from build123d import *
from OCP.BRepFilletAPI import BRepFilletAPI_MakeChamfer

# Parameters (mm, degrees)
SKETCH1_W           = 10.03
SKETCH1_H           = 7.51
BOSS_EXTRUDE1_DEPTH = 7.62
SKETCH2_W           = 2.03
SKETCH2_H           = 4.06
BOSS_EXTRUDE2_DEPTH = 0.89
CHAMFER1_SIZE       = 0.89
CHAMFER1_SIZE_2     = 0.238474781
SKETCH3_W           = 2.03
SKETCH3_H           = 4.06
CUT_EXTRUDE1_DEPTH  = 0.25
BOSS_EXTRUDE3_DEPTH = 0.28
LPATTERN1_COUNT     = 2
LPATTERN1_PITCH     = 2.54
FILLET1_R           = 0.1


with BuildPart() as part:
    # Sketch1 → Boss-Extrude1 (new body)
    with BuildSketch(Plane(origin=(0, 0, 0), x_dir=(1, 0, 0), z_dir=(0, 1, 0))):
        Rectangle(SKETCH1_W, SKETCH1_H)
    extrude(amount=BOSS_EXTRUDE1_DEPTH)

    # Sketch2 → Boss-Extrude2 (add)
    with BuildSketch(Plane(origin=(0, 7.62, 0), x_dir=(1, 0, 0), z_dir=(0, 1, 0))):
        with Locations((-1.015, 0)):
            Rectangle(SKETCH2_W, SKETCH2_H)
    extrude(amount=BOSS_EXTRUDE2_DEPTH)

    # Chamfer1
    chamfer1_edges_1 = [part.edges().sort_by_distance(p)[0] for p in [
        (-1.015, 8.51, -2.03),
    ]]
    chamfer1_side_1 = [part.faces().sort_by_distance(p)[0] for p in [
        (-1.015, 8.505230504, -2.03),
    ]]
    chamfer1_edges_2 = [part.edges().sort_by_distance(p)[0] for p in [
        (-1.015, 8.51, 2.03),
    ]]
    chamfer1_side_2 = [part.faces().sort_by_distance(p)[0] for p in [
        (-1.015, 8.505230504, 2.03),
    ]]
    chamfer1 = BRepFilletAPI_MakeChamfer(part.part.solid().wrapped)
    for e in chamfer1_edges_1:
        chamfer1.Add(CHAMFER1_SIZE - 0.0001, CHAMFER1_SIZE_2 - 0.0001, e.wrapped, chamfer1_side_1[0].wrapped)
    for e in chamfer1_edges_2:
        chamfer1.Add(CHAMFER1_SIZE - 0.0001, CHAMFER1_SIZE_2 - 0.0001, e.wrapped, chamfer1_side_2[0].wrapped)
    add(Compound.cast(chamfer1.Shape()), mode=Mode.REPLACE)  # a hair under: the kernel refuses the full size

    # Sketch3 → Cut-Extrude1 (cut)
    with BuildSketch(Plane(origin=(0, 7.62, 0), x_dir=(1, 0, 0), z_dir=(0, 1, 0))):
        with Locations((1.015, 0)):
            Rectangle(SKETCH3_W, SKETCH3_H)
    extrude(amount=-CUT_EXTRUDE1_DEPTH, mode=Mode.SUBTRACT)

    # Sketch4 → Boss-Extrude3 (add, symmetric)
    with BuildSketch(Plane.XY.offset(1.27)):
        Polygon((4.33, 0), (4, 0), (4, -1.85), (5.2, -1.85), (5.2, -1.52), (4.33, -1.52), align=None)
        Polygon((-4, -1.85), (-5.2, -1.85), (-5.2, -1.52), (-4.33, -1.52), (-4.33, 0), (-4, 0), align=None)
    boss_extrude3 = extrude(amount=BOSS_EXTRUDE3_DEPTH, both=True)

    # LPattern1: Boss-Extrude3 ×2
    with Locations(*[(0, 0, -i * LPATTERN1_PITCH) for i in range(1, LPATTERN1_COUNT)]):
        add(boss_extrude3)

    # Fillet1
    fillet1_edges = [part.edges().sort_by_distance(p)[0] for p in [
        (5.015, 7.62, 0),
        (0, 7.62, -3.755),
        (-5.015, 7.62, 0),
        (0, 7.62, 3.755),
        (-5.015, 3.81, -3.755),
        (5.015, 3.81, -3.755),
        (5.015, 3.81, 3.755),
        (-5.015, 3.81, 3.755),
    ]]
    fillet(fillet1_edges, radius=FILLET1_R)


solid = part.part
Verification items for the finished model (mm, model axes). A direction names the side the tool comes from. Give positions to 0.01 mm unless a question says otherwise; leave off trailing zeros. Order: outer loops, then holes, each group sorted by start corner. A loop starts at its lowest first (then second) coordinate and runs counter-clockwise, first axis right, second up. Notation, with made-up numbers: M 28.5,60.5 L 42.5,60.5 A33 ccw 42.5,95.5 Z; hole C -3,-30 d9. An arc over 180 degrees is marked long. Use one line per item in the form item = value. Start each with the question number.
Q1. Scan lines: line 1 along Y through (x, z) = (-3.5, -2); line 2 along X through (y, z) = (7.75, 0); line 3 along Y through (x, z) = (0.25, 1.5). Record each from-to range of solid material in increasing order. Write a range as [from, to].
Q2. Go/stop test with flat-tipped pins: pin 1 Ø2.5 at (x, z) = (-1, 1.5) entering from -Y; pin 2 Ø1.6 at (x, z) = (1, 0) entering from +Y; pin 3 Ø0.6 at (y, z) = (8, 0.5) entering from +X; pin 4 Ø1.3 at (x, y) = (-4.5, -0.5) entering from +Z (3 decimals). Record where each tip stops, or that it passes through.
Q3. Section check B-B (z = 0.75). Enter the section's corners in (x, y) (3 decimals), then the cut area to 3 significant figures.
Q4. Section check D-D (y = 5.5). Enter the section's corners in (x, z) (3 decimals).
Q5. Mould release check, pull along Z, two halves, no side actions. Record for faces 1 (the flat face through (0, 4, 3.755)), 2 (the flat face through (-5.015, 4, 0)), 3 (the flat face through (0, 8, 0)): +Z half, -Z half, draft (parallel to the pull), parting line (faces both ways), or undercut.
Q6. Section check A-A (y = -0.5). Enter the section's corners in (x, z), then the cut area to 3 significant figures.
Q7. Access from +Z, -Z, +X, -X, +Y, -Y to the whole of each face (thin tool, end or side, straight path). Record for faces 4 (the flat face through (0, 4, -3.755)), 5 (the flat face through (-2.03, 8, 0)).
Evaluation:
q1.line_1 = [0, 7.62]
q1.line_2 = [-2.03, 0]
q1.line_3 = [0, 7.37]
q2.pin_1 = 0
q2.pin_2 = 7.37
q2.pin_3 = 0
q2.pin_4 = 3.755
q3.outline = M -5.015,0 L 5.015,0 L 5.015,7.52 A0.1 ccw 4.915,7.62 L 2.03,7.62 L 2.03,7.37 L 0,7.37 L 0,8.51 L -2.03,8.51 L -2.03,7.62 L -4.915,7.62 A0.1 ccw -5.015,7.52 Z
q3.area = 77.7 mm2
q4.outline = M -5.015,-3.655 A0.1 ccw -4.915,-3.755 L 4.915,-3.755 A0.1 ccw 5.015,-3.655 L 5.015,3.655 A0.1 ccw 4.915,3.755 L -4.915,3.755 A0.1 ccw -5.015,3.655 Z
q5.face_1 = +Z half
q5.face_2 = draft
q5.face_3 = undercut
q6.outline = M -4.33,-1.55 L -4,-1.55 L -4,-0.99 L -4.33,-0.99 Z; M -4.33,0.99 L -4,0.99 L -4,1.55 L -4.33,1.55 Z; M 4,-1.55 L 4.33,-1.55 L 4.33,-0.99 L 4,-0.99 Z; M 4,0.99 L 4.33,0.99 L 4.33,1.55 L 4,1.55 Z
q6.area = 0.739 mm2
q7.face_4 = -Z, +X, -X, +Y, -Y
q7.face_5 = +Z, -Z, -X, +Y
